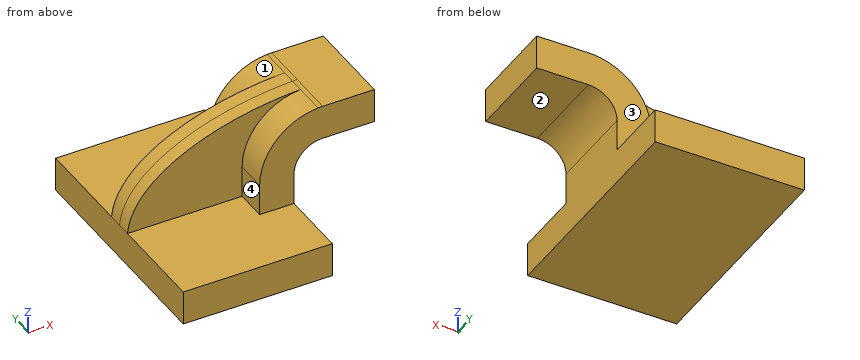
from build123d import *

# Parameters (mm, degrees)
F1_DEPTH = 63.5
F2_DEPTH = 25.4
F0_W     = 25.4
F0_H     = 19.05
F3_DEPTH = 25.4
F4_DEPTH = 7.9375


with BuildPart() as f1:
    # F0 (on Front) → F1 (new body, symmetric)
    with BuildSketch(Plane.XZ):
        Polygon((-41.275, 9.525), (-41.275, -9.525), (41.275, -9.525), (41.275, 9.525), (22.225, 9.525), align=None)
    extrude(amount=F1_DEPTH, both=True)

    # F0 (on Front) → F2 (join, symmetric)
    with BuildSketch(Plane.XZ):
        with BuildLine():
            Line((22.225, 9.525), (41.275, 9.525))
            Line((41.275, 9.525), (41.275, 27.0002))
            ThreePointArc((41.275, 27.0002), (45.92468, 38.22552), (57.15, 42.8752))
            Line((57.15, 42.8752), (60.325, 42.8752))
            Line((60.325, 42.8752), (60.325, 61.9252))
            Line((60.325, 61.9252), (57.15, 61.9252))
            add(Edge.make_bspline(
                [(54.618109, 61.833304), (55.461271, 61.86945), (56.305306, 61.900096), (57.15, 61.9252)],
                knots=[109.579831, 109.579831, 109.579831, 109.579831, 111.504536, 111.504536, 111.504536, 111.504536], degree=3))
            ThreePointArc((54.618109, 61.833304), (31.574798, 50.783906), (22.225, 27.0002))
            Line((22.225, 27.0002), (22.225, 9.525))
        make_face()
    extrude(amount=F2_DEPTH, both=True)

    # F0 (on Front) → F3 (join, symmetric)
    with BuildSketch(Plane.XZ):
        with Locations((73.025, 52.4002)):
            Rectangle(F0_W, F0_H)
    extrude(amount=F3_DEPTH, both=True)

    # F0 (on Front) → F4 (join, symmetric)
    with BuildSketch(Plane.XZ):
        with BuildLine():
            add(Edge.make_bspline(
                [(-41.275, 9.525), (-38.560078, 39.886518), (6.614079, 59.775381), (54.618109, 61.833304)],
                knots=[0, 0, 0, 0, 109.579831, 109.579831, 109.579831, 109.579831], degree=3))
            Line((-41.275, 9.525), (22.225, 9.525))
            Line((22.225, 9.525), (22.225, 27.0002))
            ThreePointArc((22.225, 27.0002), (31.574798, 50.783906), (54.618109, 61.833304))
        make_face()
    extrude(amount=F4_DEPTH, both=True)


solid = f1.part
Design review of the part built by this model. Coordinates are the model's own, in mm. Face numbers are marked on the shaded views. A direction names the side the tool comes from. Coordinates: 2 decimals unless noted, no trailing zeros. Order: outer loops, then holes, each group sorted by start corner. A loop starts at its lowest first (then second) coordinate and runs counter-clockwise, first axis right, second up. Notation, with made-up numbers: (84.5, -1) - (126.5, -1) arc R16 cw to (126.5, 11) - close; hole circle Ø11 at (46, 5.5). An arc over 180 degrees is marked (long way). Put each result on its own line as item: value.
1) Wall thickness on L1, parallel to Z at x = 1, y = 23.5 (3 decimals); L2, parallel to X at y = 51.5, z = 2 (3 decimals); L3, parallel to Y at x = 46, z = 51: over which ranges is each line inside the solid? List them lowest first. Write a range as from..to.
Response values:
L1: z = -9.525..9.525
L2: x = -41.275..41.275
L3: y = -25.4..25.4
2) Insertion check: P1, Ø18.5, axis at y = -23.5, z = 4, coming from the +X side (3 decimals); P2, Ø10, axis at y = 34.5, z = 42, coming from the -X side; P3, Ø23, axis at x = 72, y = 5, coming from the -Z side; P4, Ø5, axis at y = -19, z = 17.5, coming from the -X side (3 decimals). Each pin has a flat end and moves straight along its axis. Give the tip position at first contact, or say it passes through.
Response values:
P1: stops at x = 41.275
P2: passes through
P3: stops at z = 42.88
P4: stops at x = 22.225
3) Tool access review of the marked faces 1, 2, 3 and 4: name each direction out of +Z, -Z, +X, -X, +Y, -Y from which nothing blocks a thin tool from reaching the whole face with its end or side.
Response values:
face 1: +Z, -X, +Y
face 2: -Z, +X, +Y, -Y
face 3: +Z, +X, -X, +Y
face 4: +Z, -X, -Y
4) Take a section at B-B, the plane y = 44.5. Give the boundary of the cut face in (x, z) (3 decimals), and give its area (3 significant figures).
Response values:
outline: (-41.275, -9.525) - (41.275, -9.525) - (41.275, 9.525) - (-41.275, 9.525) - close
area: 1,570 mm²
5) Take a section at A-A, the plane z = -2. Give the boundary of the cut face in (x, y) (3 decimals).
Response values:
outline: (-41.275, -63.5) - (41.275, -63.5) - (41.275, 63.5) - (-41.275, 63.5) - close
